Drawing for the job (mm, zero at the part's lowest x, y, z). A direction names the side the tool comes from. Give positions to 0.01 mm unless a question says otherwise; leave off trailing zeros. Loops run counter-clockwise (first coordinate to the right, second up) from the corner with the lowest first, then second, coordinate; pieces in that order, holes last.
1) Two-plate mould, pull along Z, no slides. Class the marked faces 1, 2 and 3: +Z half, -Z half, draft (parallel to the pull), parting line (faces both ways), or undercut.
2) Band-saw the part on D-D on x = 88. List the corners of the cut face in (y, z).
3) Wall check: line 1 (Z direction, x = 56, y = 1); line 2 (X direction, y = 2.5, z = 33.5); line 3 (Y direction, x = 61, z = 37). Give the ranges that are in metal, low to high.
4) Band-saw the part on A-A on y = 21.25. List the corners of the cut face in (x, z), then the cut area to 3 significant figures.
5) Flat gauge pins, fed straight in: P1, Ø4, axis at x = 118, y = 10.5, coming from the -Z side; P2, Ø4, axis at x = 53, y = 3, coming from the -Z side; P3, Ø2.5, axis at y = 16.5, z = 41.5, coming from the -X side; P4, Ø4, axis at x = 78, z = 37, coming from the +Y side. Where does each tip first touch, or does it go through?
6) Band-saw the part on C-C on z = 8. List the corners of the cut face in (x, y), then the cut area to 3 significant figures.
7) Band-saw the part on B-B on x = 42.5. List the corners of the cut face in (y, z), then the cut area to 3 significant figures.
8) 3-axis set-ups, long thin cutter, end or side, ignore diameter. For the marked faces 4 and 5: which of +Z, -Z, +X, -X, +Y, -Y reach the whole face in a straight line?
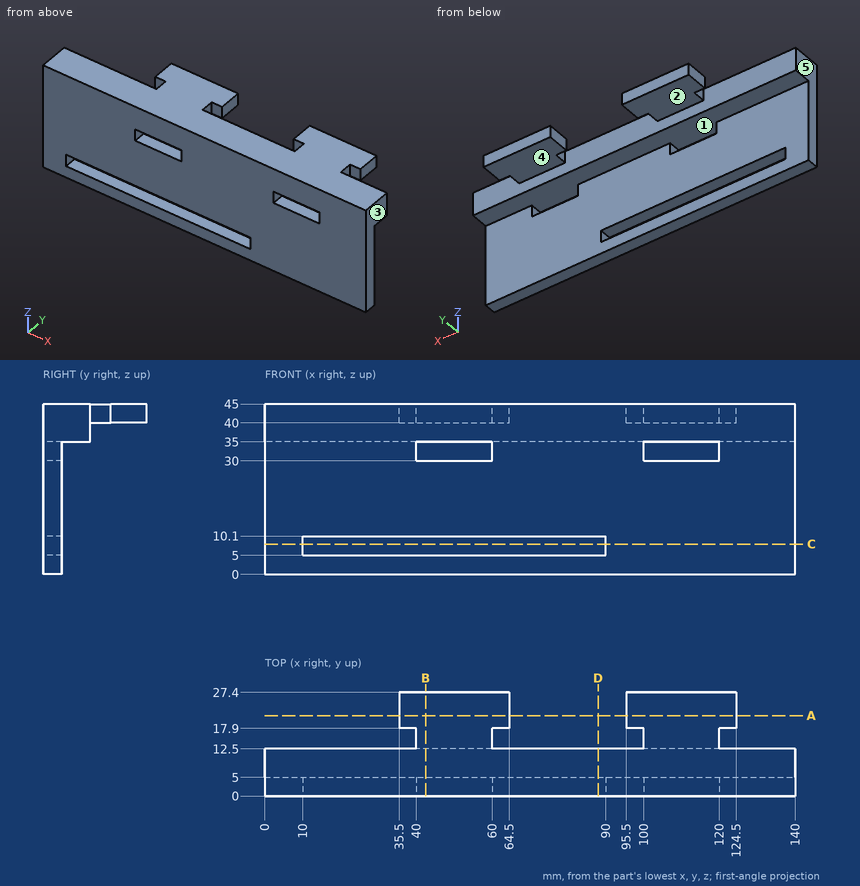
Findings below:
1. face 1: undercut
1. face 2: -Z half
1. face 3: draft
2. outline: (0, 0) - (5, 0) - (5, 5) - (0, 5) - close; (0, 10.1) - (5, 10.1) - (5, 35) - (12.5, 35) - (12.5, 45) - (0, 45) - close
3. line 1: z = 0 to 5, 10.1 to 30, 35 to 45
3. line 2: x = 0 to 40, 60 to 100, 120 to 140
3. line 3: y = 0 to 12.5
4. outline: (35.5, 40) - (64.5, 40) - (64.5, 45) - (35.5, 45) - close; (95.5, 40) - (124.5, 40) - (124.5, 45) - (95.5, 45) - close
4. area: 290 mm2
5. P1: stops at z = 35
5. P2: stops at z = 0
5. P3: stops at x = 40
5. P4: stops at y = 12.5
6. outline: (0, 0) - (10, 0) - (10, 5) - (0, 5) - close; (90, 0) - (140, 0) - (140, 5) - (90, 5) - close
6. area: 300 mm2
7. outline: (0, 0) - (5, 0) - (5, 5) - (0, 5) - close; (0, 10.1) - (5, 10.1) - (5, 30) - (0, 30) - close; (0, 35) - (12.5, 35) - (12.5, 40) - (27.4, 40) - (27.4, 45) - (0, 45) - close
7. area: 324 mm2
8. face 4: -Z, +X, -X, +Y
8. face 5: +Z, -Z, -X, +Y, -Y
